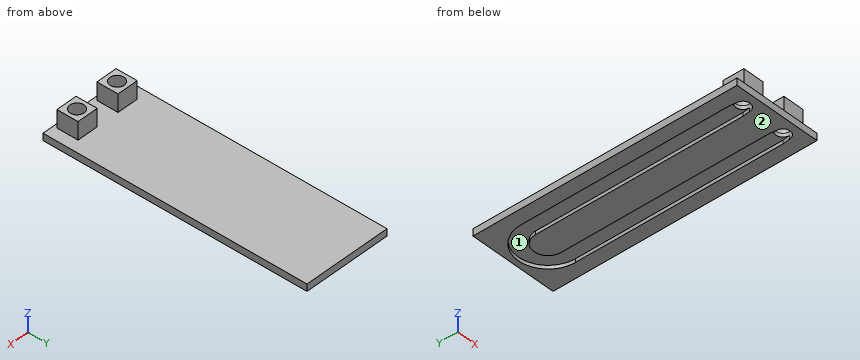
from build123d import *

# Parameters (mm, degrees)
F0_W     = 25
F0_H     = 75
F3_DEPTH = 2
F4_DEPTH = 1
F7_DEPTH = 7
F6_W     = 6
F6_H     = 6
F6_R     = 2
F8_DEPTH = 5


with BuildPart() as f3:
    # F0 (on Top) → F3 (new body)
    with BuildSketch(Plane.XY):
        with Locations((-31.788486, -12.391831)):
            Rectangle(F0_W, F0_H)
    extrude(amount=F3_DEPTH)

    # F1 (on face) → F4 (cut)
    with BuildSketch(Plane.XY):
        with BuildLine():
            ThreePointArc((-27.538486, -45.891831), (-25.538486, -47.891831), (-23.538486, -45.891831))
            ThreePointArc((-23.538486, -45.891831), (-25.538486, -43.891831), (-27.538486, -45.891831))
        make_face()
        with BuildLine():
            ThreePointArc((-27.538486, -45.891831), (-25.538486, -43.891831), (-23.538486, -45.891831))
            Line((-23.538486, -45.891831), (-23.288486, -43.891831))
            Line((-23.288486, -43.891831), (-23.288486, 15.108169))
            ThreePointArc((-23.288486, 15.108169), (-31.788486, 23.608169), (-40.288486, 15.108169))
            Line((-40.288486, 15.108169), (-40.288486, -43.891831))
            Line((-40.288486, -43.891831), (-40.038486, -45.891831))
            ThreePointArc((-40.038486, -45.891831), (-38.038486, -43.891831), (-36.038486, -45.891831))
            Line((-36.038486, -45.891831), (-35.788486, -43.891831))
            Line((-35.788486, -43.891831), (-35.788486, 15.108169))
            ThreePointArc((-35.788486, 15.108169), (-31.788486, 19.108169), (-27.788486, 15.108169))
            Line((-27.788486, 15.108169), (-27.788486, -43.891831))
            Line((-27.788486, -43.891831), (-27.538486, -45.891831))
        make_face()
        with BuildLine():
            ThreePointArc((-36.038486, -45.891831), (-38.038486, -43.891831), (-40.038486, -45.891831))
            ThreePointArc((-40.038486, -45.891831), (-38.038486, -47.891831), (-36.038486, -45.891831))
        make_face()
    extrude(amount=F4_DEPTH, mode=Mode.SUBTRACT)

    # F1 (on face) → F7 (cut)
    with BuildSketch(Plane.XY):
        with BuildLine():
            ThreePointArc((-36.038486, -45.891831), (-38.038486, -43.891831), (-40.038486, -45.891831))
            ThreePointArc((-40.038486, -45.891831), (-38.038486, -47.891831), (-36.038486, -45.891831))
        make_face()
        with BuildLine():
            ThreePointArc((-27.538486, -45.891831), (-25.538486, -47.891831), (-23.538486, -45.891831))
            ThreePointArc((-23.538486, -45.891831), (-25.538486, -43.891831), (-27.538486, -45.891831))
        make_face()
    extrude(amount=F7_DEPTH, mode=Mode.SUBTRACT)

    # F6 (on face) → F8 (join)
    with BuildSketch(Plane.XY.offset(2)):
        with Locations((-38.038486, -45.891831)):
            Rectangle(F6_W, F6_H)
        with Locations((-38.038486, -45.891831)):
            Circle(F6_R, mode=Mode.SUBTRACT)
        with Locations((-25.538486, -45.891831)):
            Rectangle(F6_W, F6_H)
        with Locations((-25.538486, -45.891831)):
            Circle(F6_R, mode=Mode.SUBTRACT)
    extrude(amount=F8_DEPTH)


solid = f3.part
Model file for the job. Use its own axes, mm. Face numbers are marked on the shaded views. Give positions to 0.01 mm unless a question says otherwise; leave off trailing zeros. Order: outer loops, then holes, each group sorted by start corner. A loop starts at its lowest first (then second) coordinate and runs counter-clockwise, first axis right, second up. Notation, with made-up numbers: M -25,7 L 10,7 A18 ccw 10,33 Z; hole C -40,-13 d3. An arc over 180 degrees is marked long. Put each result on its own line as item: value. Start each with the question number.
(1) Pin check, flat tips, straight feed: pin 1 Ø3 at (x, y) = (-31.5, 2) entering from +Z; pin 2 Ø5 at (x, y) = (-25.54, -45.89) entering from -Z; pin 3 Ø1.5 at (x, z) = (-36, 4.5) entering from +Y; pin 4 Ø4 at (y, z) = (-46, 4.5) entering from +X. Stop position of each tip, or through.
(2) Pull direction Y, two halves, no side cores. Call the marked faces 1 and 2: released by +Y, released by -Y, zero draft, split by the parting line, or undercut.
(3) Band-saw the part on A-A on z = 3.5. Give the cut face in (x, y).
(4) Band-saw the part on B-B on x = -36.75. Give the cut face in (y, z).
(5) Drill centre lines: L1, parallel to Z at x = -27.25, y = -42.5; L2, parallel to Y at x = -27.75, z = 4; L3, parallel to Z at x = -23, y = -1. Where is each one in solid material? Low to high. Write a range as [from, to].
(6) Band-saw the part on C-C on y = -38.5. Give the cut face in (x, z), then the cut area to 3 significant figures.
(7) Band-saw the part on D-D on x = -32.25. Give the cut face in (y, z), then the cut area to 3 significant figures.
Results below:
1. pin 1: stops at z = 2
1. pin 2: stops at z = 0
1. pin 3: stops at y = -42.89
1. pin 4: stops at x = -22.54
2. face 1: undercut
2. face 2: zero draft
3. outline: M -41.04,-48.89 L -35.04,-48.89 L -35.04,-42.89 L -41.04,-42.89 Z; M -28.54,-48.89 L -22.54,-48.89 L -22.54,-42.89 L -28.54,-42.89 Z; hole C -38.04,-45.89 d4; hole C -25.54,-45.89 d4
4. outline: M -49.89,0 L -47.42,0 L -47.42,7 L -48.89,7 L -48.89,2 L -49.89,2 Z; M -44.36,1 L 22.01,1 L 22.01,0 L 25.11,0 L 25.11,2 L -42.89,2 L -42.89,7 L -44.36,7 Z
5. L1: z = [1, 2]
5. L2: y = [-48.89, -42.89]
5. L3: z = [0, 2]
6. outline: M -44.29,0 L -40.29,0 L -40.29,1 L -35.79,1 L -35.79,0 L -27.79,0 L -27.79,1 L -23.29,1 L -23.29,0 L -19.29,0 L -19.29,2 L -44.29,2 Z
6. area: 41.0 mm2
7. outline: M -49.89,0 L 19.08,0 L 19.08,1 L 23.6,1 L 23.6,0 L 25.11,0 L 25.11,2 L -49.89,2 Z
7. area: 145 mm2
